The listing builds one solid part. Answer for the finished solid, in the listing's coordinates (mm). A direction names the side the tool comes from. Give positions to 0.01 mm unless a question says otherwise; leave off trailing zeros. Write each loop counter-clockwise with the first axis right and the second up, starting at its lowest first coordinate (ties: lowest second). Pieces come first, ordered by that corner, then holes. Notation, with made-up numbers: M 74,14 L 109,14 A11 ccw 109,18 Z; hole C 14.5,58.5 d3. An arc over 180 degrees is marked long. Answer as a JSON object with one key per item and string values.
Autodesk Inventor part; units mm, degrees
ref_plane "YZ Plane" through (0, 0, 0) normal (1, 0, 0) x (0, 1, 0)
ref_plane "XZ Plane" through (0, 0, 0) normal (0, 1, 0) x (-1, 0, 0)
ref_plane "Work Plane1" through (0, 0, 44.5407) normal (0, 0, 1) x (1, 0, 0)
sketch "Sketch2" plane through (0, 0, 44.5407) normal (0, 0, 1) x (1, 0, 0)
  line L0 (0, 34.026) -> (32.3607, 10.5146)
  line L1 (32.3607, 10.5146) -> (20, -27.5276)
  line L2 (20, -27.5276) -> (-20, -27.5276)
  line L3 (-20, -27.5276) -> (-32.3607, 10.5146)
  line L4 (-32.3607, 10.5146) -> (0, 34.026)
  point P0 (0, 0)
  point P1 (0, 0)
  dimension "d2" = 40
loft "Loft1" add profiles "Sketch2" section 2 point at (0, 0, 0)
mirror "Mirror1" about plane through (32.3607, 10.5146, 44.5407) normal (0.809017, -0.2628656, -0.5257311) of "Loft1"
mirror "Mirror2" about plane through (20, -27.5276, 44.5407) normal (0, -0.8506508, -0.5257311) of "Loft1"
mirror "Mirror3" about plane through (-20, -27.5276, 44.5407) normal (-0.809017, -0.2628656, -0.5257311) of "Loft1"
mirror "Mirror4" about plane through (-32.3607, 10.5146, 44.5407) normal (-0.5, 0.688191, -0.5257311) of "Loft1"
mirror "Mirror5" about plane through (0, 34.026, 44.5407) normal (0.5, 0.688191, -0.5257311) of "Loft1"
mirror "Mirror6" about plane through (-52.3607, -17.013, -10.5146) normal (0.309017, -0.4253254, -0.8506508) of "Loft1", "Mirror3"
mirror "Mirror7" about plane through (-52.3607, 17.013, 10.5146) normal (0, 0.5257311, -0.8506508) of "Loft1", "Mirror3"
mirror "Mirror8" about plane through (52.3607, -17.013, -10.5146) normal (0, 0.5257311, -0.8506508) of "Loft1", "Mirror1"
mirror "Mirror9" about plane through (20, 27.5276, -44.5407) normal (-0.809017, -0.2628656, -0.5257311) of "Loft1", "Mirror1", "Mirror8"
shell "Shell1" thickness 2 removed faces 9 at (-17.4536, 35.3648, 21.8566) at (0, 36.7035, -26.1889) at (21.5738, 29.6938, 26.1889) at (-6.6667, -2.1661, 44.5407) at (39.0273, -5.671, 21.8566) at (39.0273, 17.013, -14.8469) at (-4.1202, -5.671, -44.5407) at (-41.5738, 9.1759, -14.8469) at (-39.0273, -5.671, 21.8566)
sketch "Sketch3" plane through (-32.3607, -44.5407, 10.5146) normal (-0.5257311, -0.7236068, -0.4472136) x (0.809017, -0.2628656, -0.5257311)
  line L0 (-13.5363, -38.4242) -> (20, -62.7897)
  line L1 (-13.5363, -38.4242) -> (-8.0063, -42.442)
  line L2 (-1.4531, -1.2361) -> (-13.5363, -38.4242)
  line L3 (-13.5363, -38.4242) -> (-11.5295, -32.2482)
  line L4 (-13.5363, -38.4242) -> (-7.8299, -36.5701)
  circle A0 centre (-7.8299, -36.5701) radius 1.5
  point P0 (20, -27.5276)
  dimension "d8" = 6
  dimension "d9" = 54
  dimension "d10" = 108
  dimension "d11" = 3
extrude "Extrusion1" cut sketch "Sketch3" against normal through all
sketch "Sketch4" plane through (0, -55.0553, -10.5146) normal (0.5257311, -0.7236068, -0.4472136) x (0.809017, 0.2628656, 0.5257311)
  line L0 (52.3607, -38.0423) -> (53.5363, -38.4242)
  line L1 (53.5363, -38.4242) -> (50.6191, -40.5437)
  line L2 (20, -62.7897) -> (53.5363, -38.4242)
  line L3 (53.5363, -38.4242) -> (53.5363, -38.4242)
  line L4 (53.5363, -38.4242) -> (41.4531, -1.2361)
  line L5 (53.5363, -38.4242) -> (47.8299, -36.5701)
  circle A0 centre (47.8299, -36.5701) radius 1.5
  point P0 (20, -27.5276)
  dimension "d14" = 6
  dimension "d15" = 108
  dimension "d16" = 54
  dimension "d17" = 3
extrude "Extrusion2" cut sketch "Sketch4" against normal through all
equation "\"d9\" = 0.5 * d10"
properties part number "dodecahedron"
1. The mould has two halves that part along Y. Classify faces 1 (the flat face through (-25.814, -28.23, -19.101)), 2 (the cylindrical face through (49.062, -17.699, -11.078)), 3 (the flat face through (0, -26, 44.541)): released by +Y, released by -Y, zero draft, split by the parting line, or undercut.
Verdict:
{"face 1": "released by +Y", "face 2": "undercut", "face 3": "zero draft"}
2. A cutting plane is placed at C-C, the plane z = -22. Give the vertices of the cut face in (x, y).
Verdict:
{"outline": "M -45.61,-14.82 L 0,-47.96 L 45.61,-14.82 L 44.88,-12.58 L 0,-45.19 L -44.88,-12.58 Z"}
3. A cutting plane is placed at A-A, the plane y = -40. Give the vertices of the cut face in (x, z), plus the area to 3 significant figures.
Verdict:
{"outline": "M -35.66,7.05 L 0,-34.87 L 35.66,7.05 L 34.21,9.81 L 0,-30.4 L -34.21,9.81 Z; M -31.41,15.12 L 31.41,15.12 L 29.06,19.6 L -29.06,19.6 Z", "area": "583 mm2"}
4. Flat-ended cylindrical pins translate along their axes: pin 1 (4 mm diameter, centred on y = -42.5, z = 14.5, fed in from +X); pin 2 (2 mm diameter, centred on x = 26.5, z = -3.5, fed in from -Y); pin 3 (4 mm diameter, centred on x = 22.5, z = 33.5, fed in from -Y). Find the tip coordinate at first contact, or state that the pin passes through.
Verdict:
{"pin 1": "stops at x = 32.16", "pin 2": "stops at y = -41.09", "pin 3": "stops at y = -34.05"}
5. Consider line 1 along Z through (x, y) = (-10, -32.5); line 2 along X through (y, z) = (-16, -35.5); line 3 along Z through (x, y) = (-15.5, -29). Determine where each line is inside the solid, lowest interval first.
Verdict:
{"line 1": "z = -35.25 to -30.78, 30.12 to 34.6", "line 2": "x = -32.5 to -28.7, 28.7 to 32.5", "line 3": "z = -34.45 to -29.98, 37.12 to 41.6"}
6. A cutting plane is placed at D-D, the plane y = -46.5. Give the vertices of the cut face in (x, z).
Verdict:
{"outline": "M -26.33,6.6 L 0,-24.36 L 26.33,6.6 Z; hole M -18.72,2.12 L 0,-19.89 L 18.72,2.12 Z"}
7. A cutting plane is placed at B-B, the plane y = -30. Give the vertices of the cut face in (x, z).
Verdict:
{"outline": "M -42.93,-0.59 L -5.54,-44.54 L -1.74,-44.54 L -41.47,2.17 Z; M -24.15,35.12 L 24.15,35.12 L 21.8,39.6 L -21.8,39.6 Z; M 1.74,-44.54 L 5.54,-44.54 L 42.93,-0.59 L 41.47,2.17 Z"}
8. For faces 4 (the flat face through (25.81, -28.71, -18.33)), 5 (the flat face through (2.82, -40.035, 19.526)), determine the directions among +Z, -Z, +X, -X, +Y, -Y from which every point of the face is accessible in a straight line to the end or side of a thin tool.
Verdict:
{"face 4": "+Y", "face 5": "+Z, +X, -X, -Y"}
